```python
from build123d import *

# Parameters (mm, degrees)
ESBO_O1_R                = 2.7
RESSALTO_EXTRUS_O1_DEPTH = 69.4
ESBO_O2_R                = 1.95
RESSALTO_EXTRUS_O2_DEPTH = 4
RESSALTO_EXTRUS_O3_START = 4
ESBO_O3_R                = 1.95
RESSALTO_EXTRUS_O3_DEPTH = 4
ESBO_O5_W                = 3.73496988
ESBO_O5_H                = 0.75
CORTE_EXTRUS_O2_DEPTH    = 15


with BuildPart() as part:
    # Esboço1 → Ressalto-extrusão1 (new body)
    with BuildSketch(Plane.XY):
        Circle(ESBO_O1_R)
    extrude(amount=RESSALTO_EXTRUS_O1_DEPTH)

    # Esboço2 → Ressalto-extrusão2 (add)
    with BuildSketch(Plane.XY.offset(69.4)):
        Circle(ESBO_O2_R)
    extrude(amount=RESSALTO_EXTRUS_O2_DEPTH)

    # Esboço3 → Ressalto-extrusão3 (add)
    with BuildSketch(Plane(origin=(0, 0, 0), x_dir=(-1, 0, 0), z_dir=(0, 0, -1)).offset(RESSALTO_EXTRUS_O3_START)):
        with Locations(Location((0, 0, 0), (0, 0, 180))):
            Circle(ESBO_O3_R)
    extrude(amount=-RESSALTO_EXTRUS_O3_DEPTH)

    # Esboço5 → Corte-extrusão2 (cut)
    with BuildSketch(Plane.XY.offset(69.4)):
        with Locations((0, 2.325)):
            Rectangle(ESBO_O5_W, ESBO_O5_H)
    extrude(amount=-CORTE_EXTRUS_O2_DEPTH, mode=Mode.SUBTRACT)


solid = part.part
```
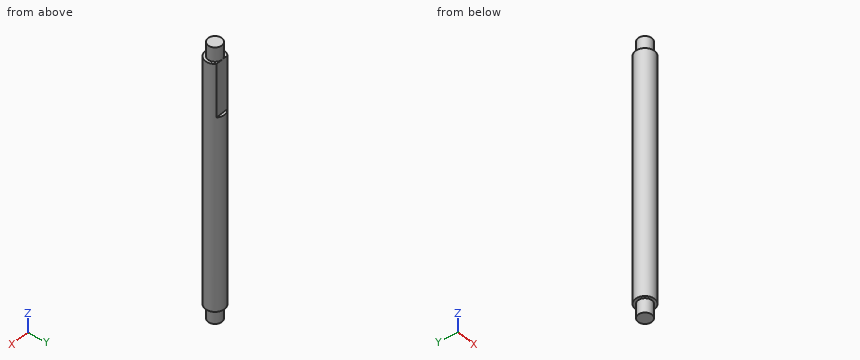
Build history of the part. All positions in model axes, mm. Round coordinates to 2 decimals unless told otherwise and drop trailing zeros. Write each loop counter-clockwise with the first axis right and the second up, starting at its lowest first coordinate (ties: lowest second). Pieces come first, ordered by that corner, then holes. Notation, with made-up numbers: (2, -13) - (46, -13) arc R14 cw to (46, 8) - close; hole circle Ø6 at (-28, 62.25). An arc over 180 degrees is marked (long way). Write each question's results on one line, items separated by ' | '. Start each with the question number.
Item 1: Wall check: L1, parallel to Z at x = -1, y = 2.05; L2, parallel to Y at x = -1.95, z = 12; L3, parallel to X at y = 1.45, z = 43. Give the ranges that are in metal, low to high. Write a range as [from, to].
Item 2: Saw through at D-D (z = 31.5). Write the cut outline in (x, y).
Item 3: Drop flat-ended pins along their axis: P1, Ø0.8, axis at x = 0, y = 2.5, coming from the +Z side; P2, Ø3, axis at x = -1, z = 64.5, coming from the +Y side; P3, Ø3, axis at y = -2, z = 28, coming from the -X side. Give the stop position or say it passes through.
Item 4: Saw through at B-B (z = 67). Write the cut outline in (x, y).
Item 5: Saw through at A-A (y = 0). Write the cut outline in (x, z), and give its area (3 significant figures).
Item 6: Saw through at C-C (x = -0.95). Write the cut outline in (y, z).
Results are:
1) L1: z = [0, 54.4] | L2: y = [-1.87, 1.87] | L3: x = [-2.28, 2.28]
2) outline: circle Ø5.4 at (0, 0)
3) P1: stops at z = 54.4 | P2: stops at y = 1.95 | P3: stops at x = -2.65
4) outline: (-1.87, 1.95) arc R2.7 ccw (long way) to (1.87, 1.95) - close
5) outline: (-2.7, 0) - (-1.95, 0) - (-1.95, -4) - (1.95, -4) - (1.95, 0) - (2.7, 0) - (2.7, 69.4) - (1.95, 69.4) - (1.95, 73.4) - (-1.95, 73.4) - (-1.95, 69.4) - (-2.7, 69.4) - close | area: 406 mm²
6) outline: (-2.53, 0) - (-1.7, 0) - (-1.7, -4) - (1.7, -4) - (1.7, 0) - (2.53, 0) - (2.53, 54.4) - (1.95, 54.4) - (1.95, 69.4) - (1.7, 69.4) - (1.7, 73.4) - (-1.7, 73.4) - (-1.7, 69.4) - (-2.53, 69.4) - close
